```python
from build123d import *

# Parameters (mm, degrees)
FILLET1_R          = 10
CUT_EXTRUDE1_START = -50
CUT_EXTRUDE1_DEPTH = 50


with BuildPart() as part:
    # Sketch1 → Revolve1 (revolve)
    with BuildSketch(Plane.XY, mode=Mode.PRIVATE) as revolve1_sk:
        Polygon((-1040, 0), (1180, 0), (1180, 50), (950, 50), (950, 177.595701724), (0, 177.595701724), (-950, 177.595701724), (-950, 50), (-1040, 50), align=None)
    revolve(revolve1_sk.sketch.rotate(Axis((-1040, 0, 0), (1, 0, 0)), 180), axis=Axis((-1040, 0, 0), (1, 0, 0)))

    # Fillet1
    fillet1_edges = [part.edges().sort_by_distance(p)[0] for p in [
        (950, 50, 0),
        (-950, 50, 0),
    ]]
    fillet(fillet1_edges, radius=FILLET1_R)

    # Sketch2 → Cut-Extrude1 (cut)
    with BuildSketch(Plane(origin=(1180, 0, 0), x_dir=(0, 0, -1), z_dir=(1, 0, 0)).offset(CUT_EXTRUDE1_START)):
        with BuildLine():
            ThreePointArc((14, 48), (0, 50), (-14, 48))
            Line((-14, 48), (-14, 45.4))
            Line((-14, 45.4), (14, 45.4))
            Line((14, 45.4), (14, 48))
        make_face()
    extrude(amount=CUT_EXTRUDE1_DEPTH, mode=Mode.SUBTRACT)


solid = part.part
```
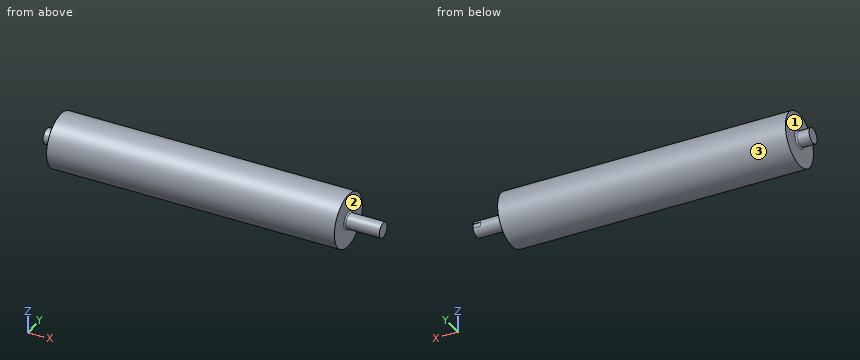
Geometry check sheet. Reference: the model listing, model coordinates, mm. Face numbers are marked on the shaded views. A direction names the side the tool comes from. Round coordinates to 2 decimals unless told otherwise and drop trailing zeros. Order: outer loops, then holes, each group sorted by start corner. A loop starts at its lowest first (then second) coordinate and runs counter-clockwise, first axis right, second up. Notation, with made-up numbers: (69, 67) - (86, 67) arc R29 ccw to (86, 106) - close; hole circle Ø8 at (-34.75, 70.25). An arc over 180 degrees is marked (long way). Use a Markdown table: item, result. Add a question column.
(1) Sectioned sample at A-A, the plane y = 0. Enter the section's corners in (x, z), and give its area (3 significant figures).
(2) Sectioned sample at D-D, the plane y = -85. Enter the section's corners in (x, z), and give its area (3 significant figures).
(3) Sectioned sample at C-C, the plane z = 110.5. Enter the section's corners in (x, y).
(4) Tool access check on the marked faces 1, 2 and 3. Record the directions out of +Z, -Z, +X, -X, +Y, -Y that give a thin tool (end or side, any length) a straight path to the whole face; none if there is none.
(5) Sectioned sample at B-B, the plane x = 515. Enter the section's corners in (y, z), and give its area (3 significant figures).
(6) Material ranges on line 1 along X through (y, z) = (125.5, 119.5); line 2 along Z through (x, y) = (532, -91.5); line 3 along Z through (x, y) = (900, -29.5), recorded low to high. Write a range as [from, to].
(7) Depth check by flat-ended pin: pin 1 (3 mm diameter, centred on y = -134, z = -39, fed in from +X); pin 2 (2 mm diameter, centred on y = 60, z = -67.5, fed in from -X); pin 3 (4 mm diameter, centred on x = 685, z = -109, fed in from -Y). Enter the tip coordinate at first touch or a pass-through.
Answers below:
| question | item | result |
|---|---|---|
| 1 | outline | (-1040, -50) - (-960, -50) arc R10 cw to (-950, -60) - (-950, -177.6) - (950, -177.6) - (950, -60) arc R10 cw to (960, -50) - (1180, -50) - (1180, 50) - (960, 50) arc R10 cw to (950, 60) - (950, 177.6) - (-950, 177.6) - (-950, 60) arc R10 cw to (-960, 50) - (-1040, 50) - close |
| 1 | area | 707,000 mm² |
| 2 | outline | (-950, -155.93) - (950, -155.93) - (950, 155.93) - (-950, 155.93) - close |
| 2 | area | 593,000 mm² |
| 3 | outline | (-950, -139.03) - (950, -139.03) - (950, 139.03) - (-950, 139.03) - close |
| 4 | face 1 | -X |
| 4 | face 2 | +X |
| 4 | face 3 | +X, -X |
| 5 | outline | circle Ø355.19 at (0, 0) |
| 5 | area | 99,100 mm² |
| 6 | line 1 | [-950, 950] |
| 6 | line 2 | [-152.21, 152.21] |
| 6 | line 3 | [-175.13, 175.13] |
| 7 | pin 1 | x = 950 |
| 7 | pin 2 | x = -950 |
| 7 | pin 3 | y = -141.74 |
